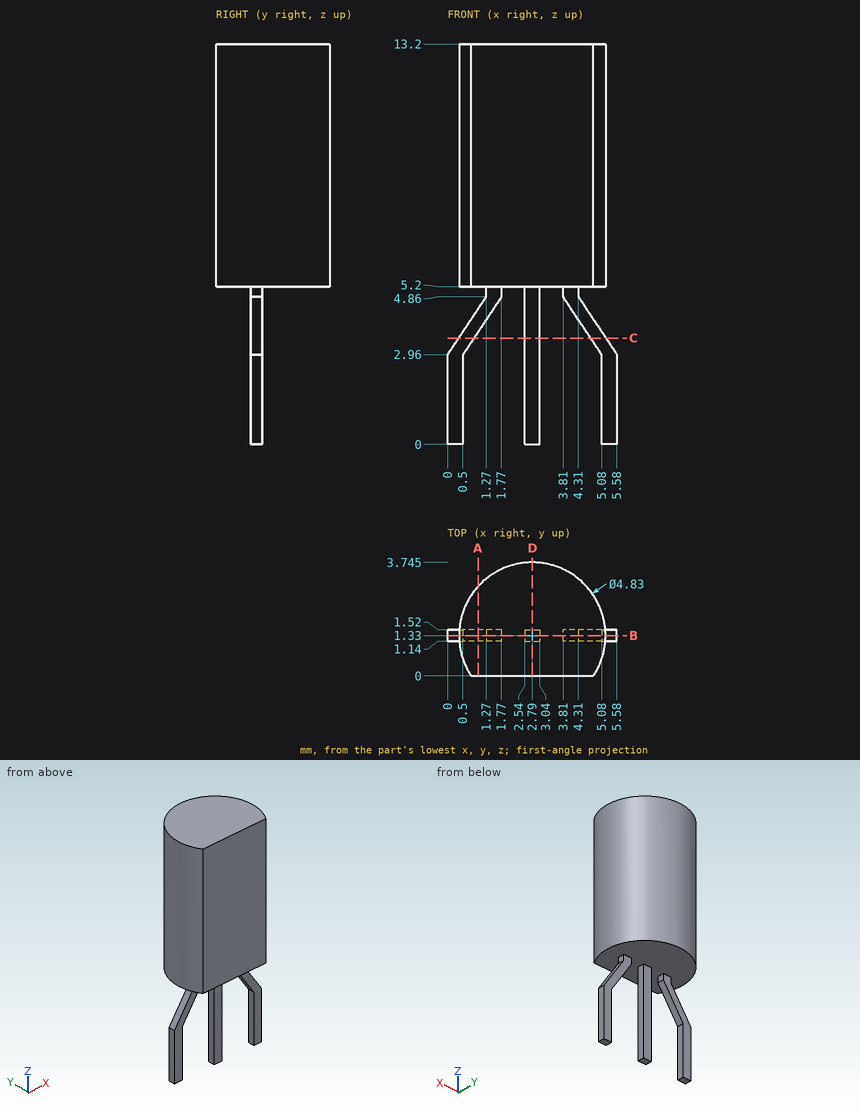
Here's the drawing with two shaded views (mm, measured from the low corner). I have some questions. Coordinates: 2 decimals unless noted, no trailing zeros. Loops run counter-clockwise (first coordinate to the right, second up) from the corner with the lowest first, then second, coordinate; pieces in that order, holes last. Notation, with made-up numbers: M 51,16 L 105,16 A18 cw 105,46 Z; hole C 52.5,14 d3. An arc over 180 degrees is marked long. Return JSON: item names as keys, results as strings. Group by question number.
Item 1: Imagine slicing it at B-B (y = 1.33). Please give me the cut outline in (x, z) (3 decimals).
Item 2: If I drill on L1, parallel to Z at x = 4.25, y = 1; L2, parallel to Y at x = 1.05, z = 4; L3, parallel to Z at x = 4.8, y = 1.2, over which ranges is the centre line in solid material (lowest first)? Write a range as from..to.
Item 3: Imagine slicing it at D-D (x = 2.79). Please give me the cut outline in (y, z) (3 decimals).
Item 4: Imagine slicing it at A-A (x = 1). Please give me the cut outline in (y, z), and give its area (3 significant figures).
Item 5: I'm going to push flat-ended pins straight in: pin 1 Ø1.1 at (x, y) = (2, 2.5) entering from -Z; pin 2 Ø1 at (y, z) = (1.5, 6.5) entering from +X (3 decimals); pin 3 Ø0.5 at (x, z) = (1, 3) entering from +Y; pin 4 Ø0.9 at (x, z) = (5, 3.5) entering from +Y. Where does each tip first touch, or does it pass through?
Item 6: Imagine slicing it at C-C (z = 3.5). Please give me the cut outline in (x, y).
Verdict:
{
 "1": {"outline": "M 0,0 L 0.5,0 L 0.5,2.96 L 1.77,4.86 L 1.77,5.2 L 2.54,5.2 L 2.54,0 L 3.04,0 L 3.04,5.2 L 3.81,5.2 L 3.81,4.86 L 5.08,2.96 L 5.08,0 L 5.58,0 L 5.58,2.96 L 4.31,4.86 L 4.31,5.2 L 5.205,5.2 L 5.205,13.2 L 0.375,13.2 L 0.375,5.2 L 1.27,5.2 L 1.27,4.86 L 0,2.96 Z"},
 "2": {"L1": "z = 5.2..13.2", "L2": "y = 1.14..1.52", "L3": "z = 3.38..4.13, 5.2..13.2"},
 "3": {"outline": "M 0,5.2 L 1.14,5.2 L 1.14,0 L 1.52,0 L 1.52,5.2 L 3.745,5.2 L 3.745,13.2 L 0,13.2 Z"},
 "4": {"outline": "M 0,5.2 L 2.95,5.2 L 2.95,13.2 L 0,13.2 Z; M 1.14,3.71 L 1.52,3.71 L 1.52,4.46 L 1.14,4.46 Z", "area": "23.9 mm^2"},
 "5": {"pin 1": "stops at z = 5.2", "pin 2": "stops at x = 5.205", "pin 3": "passes through", "pin 4": "stops at y = 1.52"},
 "6": {"outline": "M 0.36,1.14 L 0.86,1.14 L 0.86,1.52 L 0.36,1.52 Z; M 2.54,1.14 L 3.04,1.14 L 3.04,1.52 L 2.54,1.52 Z; M 4.72,1.14 L 5.22,1.14 L 5.22,1.52 L 4.72,1.52 Z"}
}
